from build123d import *

# Parameters (mm, degrees)
PAD_DEPTH = 20


with BuildPart() as part:
    # Sketch → Pad (new body)
    with BuildSketch(Plane.XY):
        with BuildLine():
            Line((0, 0), (0, 30))
            Line((0, 30), (-5, 30))
            Line((-5, 30), (-5, 0))
            Line((-15.5, 0), (-5, 0))
            ThreePointArc((-17, 1.5), (-16.56066, 0.43934), (-15.5, 0))
            Line((-17, 1.5), (-17, 23))
            ThreePointArc((-14, 23), (-15.5, 24.5), (-17, 23))
            Line((-14, 3), (-14, 23))
            Line((-8, 3), (-14, 3))
            Line((-8, 30), (-8, 3))
            ThreePointArc((-5, 33), (-7.12132, 32.12132), (-8, 30))
            Line((3, 33), (-5, 33))
            Line((3, 0), (3, 33))
            Line((0, 0), (3, 0))
        make_face()
    extrude(amount=PAD_DEPTH)


solid = part.part
Design review of the part built by this model. Coordinates are the model's own, in mm. A direction names the side the tool comes from. Round coordinates to 2 decimals unless told otherwise and drop trailing zeros. Loops run counter-clockwise (first coordinate to the right, second up) from the corner with the lowest first, then second, coordinate; pieces in that order, holes last. Notation, with made-up numbers: (85.25, 0.25) - (121.25, 0.25) arc R33 ccw to (121.25, 39.25) - close; hole circle Ø4 at (80.25, -11). An arc over 180 degrees is marked (long way). One line per question, with ' | ' between items.
1. Draft analysis for pull direction X (two halves, no side actions). For faces 1 (the face through (-15.5, 24.5, 9.9)), 2 (the face through (3, 16, 10)), 3 (the face through (-8, 17, 10)), 4 (the face through (-7.1, 32.14, 9.86)), state which applies: released by +X, released by -X, zero draft, split by the parting line, or undercut.
Results are:
face 1: undercut | face 2: released by +X | face 3: undercut | face 4: released by -X
2. For L1, parallel to X at y = 6.5, z = 2.5; L2, parallel to X at y = 28, z = 15; L3, parallel to X at y = 24, z = 13, list the stretches that pass through material, from the lowest coordinate up. Write a range as [from, to].
Results are:
L1: x = [-17, -14], [-8, -5], [0, 3] | L2: x = [-8, -5], [0, 3] | L3: x = [-16.62, -14.38], [-8, -5], [0, 3]
3. Clearance check with flat-ended pins moving along their axes: P1, Ø1.8, axis at x = -11.5, z = 6.5, coming from the +Y side; P2, Ø8, axis at x = -9.5, z = 6, coming from the +Y side. State where each tip first meets the part, or that it passes through.
Results are:
P1: stops at y = 3 | P2: stops at y = 32.96
4. We need section A-A, the plane y = 4.5. State the section outline as (x, z) points.
Results are:
outline: (-17, 0) - (-14, 0) - (-14, 20) - (-17, 20) - close; (-8, 0) - (-5, 0) - (-5, 20) - (-8, 20) - close; (0, 0) - (3, 0) - (3, 20) - (0, 20) - close
5. We need section D-D, the plane x = -10.5. State the section outline as (y, z) points, and give its area (3 significant figures).
Results are:
outline: (0, 0) - (3, 0) - (3, 20) - (0, 20) - close | area: 60.0 mm²
6. We need section B-B, the plane z = 14.5. State the section outline as (x, y) points.
Results are:
outline: (-17, 1.5) arc R1.5 ccw to (-15.5, 0) - (-5, 0) - (-5, 30) - (0, 30) - (0, 0) - (3, 0) - (3, 33) - (-5, 33) arc R3 ccw to (-8, 30) - (-8, 3) - (-14, 3) - (-14, 23) arc R1.5 ccw to (-17, 23) - close
7. We need section C-C, the plane y = 29. State the section outline as (x, z) points.
Results are:
outline: (-8, 0) - (-5, 0) - (-5, 20) - (-8, 20) - close; (0, 0) - (3, 0) - (3, 20) - (0, 20) - close
8. For faces 5 (the face through (0, 15, 10)), 6 (the face through (-11, 3, 10)), 7 (the face through (-10, 0, 10)), list the 3-axis set-ups (+Z, -Z, +X, -X, +Y, -Y) from which the entire face can be reached by the end or side of a thin tool; tool diameter is ignored.
Results are:
face 5: +Z, -Z, -Y | face 6: +Z, -Z, +Y | face 7: +Z, -Z, +X, -X, -Y
